Read the model definition and answer for the solid it produces. Units are mm, in the model's axes. Give positions to 0.01 mm unless a question says otherwise; leave off trailing zeros. Loops run counter-clockwise (first coordinate to the right, second up) from the corner with the lowest first, then second, coordinate; pieces in that order, holes last. Notation, with made-up numbers: (43, 76) - (72, 76) arc R13 cw to (72, 88) - close; hole circle Ø2 at (-2.75, -12). An arc over 180 degrees is marked (long way). Write item = value, one per line.
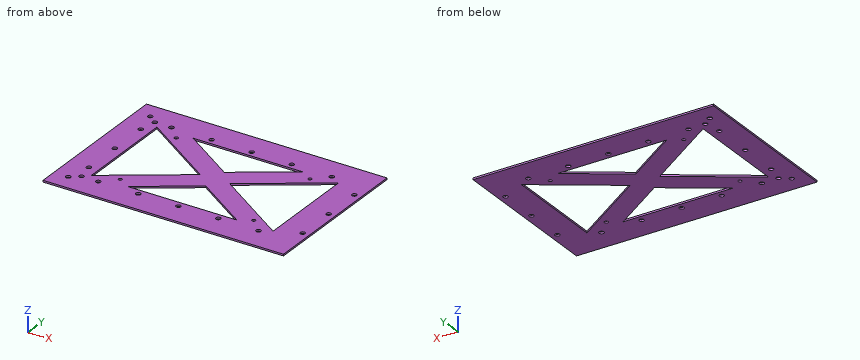
```python
from build123d import *

# Parameters (mm, degrees)
SKETCH1_W           = 228.6
SKETCH1_H           = 152.4
BOSS_EXTRUDE1_DEPTH = 1.5875
SKETCH2_R           = 2.25
CUT_EXTRUDE1_DEPTH  = 2.5875
SKETCH3_R           = 1.7
CUT_EXTRUDE2_DEPTH  = 2.5875


with BuildPart() as part:
    # Sketch1 → Boss-Extrude1 (new body)
    with BuildSketch(Plane.XY):
        Rectangle(SKETCH1_W, SKETCH1_H)
        Polygon((-52.017124101, 48.26), (52.017124101, 48.26), (0, 13.581917266), align=None, mode=Mode.SUBTRACT)
        Polygon((-86.36, 48.26), (-86.36, -48.26), (-13.97, 0), align=None, mode=Mode.SUBTRACT)
        Polygon((0, -13.581917266), (-52.017124101, -48.26), (52.017124101, -48.26), align=None, mode=Mode.SUBTRACT)
        Polygon((13.97, 0), (86.36, 48.26), (86.36, -48.26), align=None, mode=Mode.SUBTRACT)
    extrude(amount=BOSS_EXTRUDE1_DEPTH)

    # Sketch2 → Cut-Extrude1 (cut, through all)
    with BuildSketch(Plane.XY.offset(1.5875)):
        with Locations((-100.541666667, 60.325)):
            Circle(SKETCH2_R)
        with Locations((-92.075, 53.975)):
            Circle(SKETCH2_R)
        with Locations((-95.255, 38.1)):
            Circle(SKETCH2_R)
        with Locations((-95.255, 0)):
            Circle(SKETCH2_R)
        with Locations((-95.255, -38.1)):
            Circle(SKETCH2_R)
        with Locations((-92.075, -53.975)):
            Circle(SKETCH2_R)
        with Locations((-100.541666667, -60.325)):
            Circle(SKETCH2_R)
        with Locations((107.95, 38.1)):
            Circle(SKETCH2_R)
        with Locations((107.95, 0)):
            Circle(SKETCH2_R)
        with Locations((107.95, -38.1)):
            Circle(SKETCH2_R)
        with Locations((-76.2, 53.975)):
            Circle(SKETCH2_R)
        with Locations((-76.2, -53.975)):
            Circle(SKETCH2_R)
        with Locations((-38.1, -53.975)):
            Circle(SKETCH2_R)
        with Locations((-38.1, 53.975)):
            Circle(SKETCH2_R)
        with Locations((0, -53.975)):
            Circle(SKETCH2_R)
        with Locations((0, 53.975)):
            Circle(SKETCH2_R)
        with Locations((38.1, -53.975)):
            Circle(SKETCH2_R)
        with Locations((38.1, 53.975)):
            Circle(SKETCH2_R)
        with Locations((76.2, -53.975)):
            Circle(SKETCH2_R)
        with Locations((76.2, 53.975)):
            Circle(SKETCH2_R)
    extrude(amount=-CUT_EXTRUDE1_DEPTH, mode=Mode.SUBTRACT)

    # Sketch3 → Cut-Extrude2 (cut, through all)
    with BuildSketch(Plane.XY.offset(1.5875)):
        with Locations((-63.5, 41.275)):
            Circle(SKETCH3_R)
        with Locations((63.5, 41.275)):
            Circle(SKETCH3_R)
        with Locations((-63.5, -41.275)):
            Circle(SKETCH3_R)
        with Locations((63.5, -41.275)):
            Circle(SKETCH3_R)
    extrude(amount=-CUT_EXTRUDE2_DEPTH, mode=Mode.SUBTRACT)


solid = part.part
```
1) A cutting plane is placed at A-A on x = 107.95. Determine the outline of the cut face in (y, z), then the cut area to 3 significant figures.
Output:
outline = (-76.2, 0) - (-40.35, 0) - (-40.35, 1.59) - (-76.2, 1.59) - close; (-35.85, 0) - (-2.25, 0) - (-2.25, 1.59) - (-35.85, 1.59) - close; (2.25, 0) - (35.85, 0) - (35.85, 1.59) - (2.25, 1.59) - close; (40.35, 0) - (76.2, 0) - (76.2, 1.59) - (40.35, 1.59) - close
area = 221 mm²
2) A cutting plane is placed at B-B on y = 21.5. Determine the outline of the cut face in (x, z), then the cut area to 3 significant figures.
Output:
outline = (-114.3, 0) - (-86.36, 0) - (-86.36, 1.59) - (-114.3, 1.59) - close; (-46.22, 0) - (-11.88, 0) - (-11.88, 1.59) - (-46.22, 1.59) - close; (11.88, 0) - (46.22, 0) - (46.22, 1.59) - (11.88, 1.59) - close; (86.36, 0) - (114.3, 0) - (114.3, 1.59) - (86.36, 1.59) - close
area = 198 mm²
3) Find the intervals of material crossed by probe 1 along Y at (x, z) = (107.95, 0.6); probe 2 along Y at (x, z) = (76.2, 0.65) (3 decimals); probe 3 along X at (y, z) = (-1, 0.3), in increasing order.
Output:
probe_1 = -76.2 to -40.35, -35.85 to -2.25, 2.25 to 35.85, 40.35 to 76.2
probe_2 = -76.2 to -56.225, -51.725 to -41.487, 41.487 to 51.725, 56.225 to 76.2
probe_3 = -114.3 to -97.27, -93.24 to -86.36, -15.47 to 15.47, 86.36 to 105.93, 109.97 to 114.3
4) A cutting plane is placed at D-D on x = 59.5. Determine the outline of the cut face in (y, z), then the cut area to 3 significant figures.
Output:
outline = (-76.2, 0) - (-30.35, 0) - (-30.35, 1.59) - (-76.2, 1.59) - close; (30.35, 0) - (76.2, 0) - (76.2, 1.59) - (30.35, 1.59) - close
area = 146 mm²
5) A cutting plane is placed at C-C on x = -7. Determine the outline of the cut face in (y, z), then the cut area to 3 significant figures.
Output:
outline = (-76.2, 0) - (-48.26, 0) - (-48.26, 1.59) - (-76.2, 1.59) - close; (-18.25, 0) - (18.25, 0) - (18.25, 1.59) - (-18.25, 1.59) - close; (48.26, 0) - (76.2, 0) - (76.2, 1.59) - (48.26, 1.59) - close
area = 147 mm²
